Autodesk Inventor part; units mm, degrees
ref_plane "YZ Plane" through (0, 0, 0) normal (1, 0, 0) x (0, 1, 0)
ref_plane "XZ Plane" through (0, 0, 0) normal (0, 1, 0) x (-1, 0, 0)
ref_plane "XY Plane" through (0, 0, 0) normal (0, 0, 1) x (1, 0, 0)
sketch "Boceto1" plane through (0, 0, 0) normal (0, 1, 0) x (-1, 0, 0)
  line L0 (0, 0) -> (50, 0)
  line L1 (50, 0) -> (50, -65)
  line L2 (50, -65) -> (0, -65)
  line L3 (0, -65) -> (0, 0)
  line L4 (17.7, -45) -> (32.7, -45)
  line L5 (32.7, -45) -> (32.7, -20)
  line L6 (32.7, -20) -> (17.7, -20)
  line L7 (17.7, -20) -> (17.7, -45)
  line L8 (17.7, -45) -> (32.7, -20) construction
  line L9 (32.7, -45) -> (17.7, -20) construction
  line L10 (35.7, -17) -> (35.7, -48)
  line L11 (35.7, -48) -> (14.7, -48)
  line L12 (14.7, -48) -> (14.7, -17)
  line L13 (14.7, -17) -> (35.7, -17)
  line L14 (41, -1.5) -> (9, -1.5)
  line L15 (9, -1.5) -> (9, -14)
  line L16 (9, -14) -> (41, -14)
  line L17 (41, -14) -> (41, -1.5)
  line L18 (32.7, -32.5) -> (17.7, -32.5) construction
  line L19 (41, -7.75) -> (35.5, -7.75) construction
  line L20 (35.5, -7.75) -> (14.5, -7.75) construction
  line L21 (14.5, -7.75) -> (9, -7.75) construction
  circle A0 centre (35.5, -7.75) radius 1.4
  circle A1 centre (14.5, -7.75) radius 1.4
  line L22 (41, -63.5) -> (9, -63.5)
  line L23 (9, -63.5) -> (9, -51)
  line L24 (9, -51) -> (41, -51)
  line L25 (41, -51) -> (41, -63.5)
  circle A2 centre (35.5, -57.25) radius 1.4
  circle A3 centre (14.5, -57.25) radius 1.4
  line L26 (50, -32.5) -> (43.2, -32.5) construction
  line L27 (0, -32.5) -> (6.8, -32.5)
  line L28 (45.9347, 0) -> (45.9347, -14) construction
  line L29 (43.2, -32.5) -> (43.2, -14.5) construction
  line L30 (43.2, -14.5) -> (50, -14.5) construction
  circle A4 centre (43.2, -14.5) radius 1.4
  line L31 (25.2, -20) -> (25.2, -45) construction
  circle A5 centre (7.2, -14.5) radius 1.4
  circle A6 centre (35.5, -57.25) radius 1.4
  circle A7 centre (43.2, -50.5) radius 1.4
  circle A8 centre (7.2, -50.5) radius 1.4
  line L32 (35.5, -7.75) -> (14.5, -7.75)
  point P0 (25.2, -32.5)
  point P1 (25, -14)
  point P2 (25.2, -17)
  dimension "d0" = 65
  dimension "d1" = 50
  dimension "d2" = 25
  dimension "d3" = 15
  dimension "d4" = 3
  dimension "d5" = 12.5
  dimension "d6" = 32
  dimension "d7" = 3
  dimension "d8" = 5.5
  dimension "d9" = 5.5
  dimension "d10" = 2.8
  dimension "d11" = 2.8
  dimension "d12" = 6.8
  dimension "d13" = 6.8
  dimension "d14" = 14
  dimension "d15" = 2.8
  dimension "d30" = 36
  dimension "d31" = 36
  dimension "d32" = 1.5
extrude "Extrusión1" add sketch "Boceto1" along normal blind 3 contours L10 L11 L12 L13
extrude "Extrusión2" add sketch "Boceto1" against normal blind 4 contours L0 L1 L2 L3 | L17 L16 L15 L14 | L22 L23 L24 L25
extrude "Extrusión3" add sketch "Boceto1" along normal blind 2 contours L17 L16 L15 L14 | L22 L23 L24 L25
sketch "Boceto2" plane through (0, 2, 0) normal (0, 1, 0) x (1, 0, 0)
  line L0 (-41, 1.5) -> (-9, 1.5)
  line L1 (-25, 1.5) -> (-25, 14)
  line L2 (-9, 14) -> (-41, 14)
  line L3 (-20, 1.5) -> (-30, 1.5)
  line L4 (-30, 1.5) -> (-30, 14)
  line L5 (-30, 14) -> (-20, 14)
  line L6 (-20, 14) -> (-20, 1.5)
  line L7 (-20, 1.5) -> (-30, 14) construction
  line L8 (-30, 1.5) -> (-20, 14) construction
  line L9 (-32.7, 32.5) -> (-17.7, 32.5) construction
  line L10 (-41, 63.5) -> (-9, 63.5)
  line L11 (-9, 51) -> (-41, 51)
  line L12 (-30, 63.5) -> (-30, 51)
  line L13 (-20, 51) -> (-20, 63.5)
  point P0 (0, 0)
  point P1 (-25, 7.75)
  dimension "d22" = 10
extrude "Extrusión4" cut sketch "Boceto2" against normal blind 0.75
extrude "Extrusión5" add sketch "Boceto1" against normal blind 4 contours L7 L6 L5 L4 | L10 L11 L12 L13
sketch "Boceto3" plane through (0, 3, 0) normal (0, 1, 0) x (1, 0, 0)
  line L0 (-25.2, 20) -> (-25.2, 45) construction
  line L1 (-35.7, 17) -> (-14.7, 17)
  line L2 (-25.2, 17) -> (-25.2, 48)
  line L3 (-14.7, 48) -> (-35.7, 48)
  line L4 (-24.95, 17) -> (-25.45, 17)
  line L5 (-25.45, 17) -> (-25.45, 48)
  line L6 (-25.45, 48) -> (-24.95, 48)
  line L7 (-24.95, 48) -> (-24.95, 17)
  line L8 (-24.95, 17) -> (-25.45, 48) construction
  line L9 (-25.45, 17) -> (-24.95, 48) construction
  point P0 (0, 0)
  point P1 (-25.2, 32.5)
  point P2 (-24.95, 17)
  point P3 (-24.95, 48)
  point P4 (-25.45, 17)
  dimension "d27" = 0.5
extrude "Extrusión6" cut sketch "Boceto3" against normal blind 1
sketch "Boceto4" plane through (-41, 0, -1.5) normal (0, 0, 1) x (1, 0, 0)
  line L0 (16.05, 2) -> (15.55, 2)
  line L1 (21, 1.25) -> (11, 1.25)
  line L2 (-9, 0) -> (41, 0)
  line L3 (15.55, 2) -> (15.55, 3)
fillet "Empalme1" radius 2 4 edges at (-41, 1, -51) (-9, 1, -51) (-9, 1, -14) (-41, 1, -14)
equation "\"d9\" = d8"
equation "\"d13\" = d12"
properties part number "Molde 1FBR 1.0mm"
For this review, take the finished solid that the model builds, in its own axes (mm). A direction names the side the tool comes from. Round coordinates to 2 decimals unless told otherwise and drop trailing zeros. Loops run counter-clockwise (first coordinate to the right, second up) from the corner with the lowest first, then second, coordinate; pieces in that order, holes last. Notation, with made-up numbers: (-19, -35.5) - (6, -35.5) arc R21 ccw to (6, -14.5) - close; hole circle Ø11 at (-31, 13.5). An arc over 180 degrees is marked (long way). One line per question, with ' | ' between items.
Q1. Take a section at A-A (z = -57.25). Give the boundary of the cut face in (x, y).
Taken from the geometry:
outline: (-50, -4) - (-36.9, -4) - (-36.9, 2) - (-41, 2) - (-41, 0) - (-50, 0) - close; (-34.1, -4) - (-15.9, -4) - (-15.9, 2) - (-20, 2) - (-20, 1.25) - (-30, 1.25) - (-30, 2) - (-34.1, 2) - close; (-13.1, -4) - (0, -4) - (0, 0) - (-9, 0) - (-9, 2) - (-13.1, 2) - close
Q2. Take a section at B-B (y = -2.25). State how many separate pieces and enclosed holes the cut face has, and give its area (3 significant figures).
Taken from the geometry:
separate pieces: 1 | enclosed holes: 8 | area: 3,200 mm²
Q3. Take a section at C-C (x = -27). Give the boundary of the cut face in (y, z), and give its area (3 significant figures).
Taken from the geometry:
outline: (-4, -65) - (0, -65) - (0, -63.5) - (1.25, -63.5) - (1.25, -51) - (0, -51) - (0, -48) - (3, -48) - (3, -45) - (0, -45) - (0, -20) - (3, -20) - (3, -17) - (0, -17) - (0, -14) - (1.25, -14) - (1.25, -1.5) - (0, -1.5) - (0, 0) - (-4, 0) - close | area: 309 mm²
Q4. For pin 1 (1.6 mm diameter, centred on x = -18, y = 1, fed in from -Z); pin 2 (1.5 mm diameter, centred on y = 1.5, z = -30, fed in from -X); pin 3 (3.5 mm diameter, centred on x = -13.5, z = -9.5, fed in from +Y); pin 4 (4 mm diameter, centred on y = 1.5, z = -55, fed in from -X), all flat-tipped, find the tip position at first contact; note any pin that passes through.
Taken from the geometry:
pin 1: stops at z = -63.5 | pin 2: stops at x = -35.7 | pin 3: stops at y = 2 | pin 4: stops at x = -50
Q5. The part is to be moulded in two halves that separate along X. For faces 1 (the cylindrical face through (-7.95, -1.97, -13.32)), 2 (the flat face through (-35, 2, -6)), 3 (the cylindrical face through (-9.6, 1.01, -51.57)), say which applies: released by +X, released by -X, zero draft, split by the parting line, or undercut.
Taken from the geometry:
face 1: undercut | face 2: zero draft | face 3: released by +X
Q6. Take a section at D-D (z = -29.5). Give the boundary of the cut face in (x, y).
Taken from the geometry:
outline: (-50, -4) - (0, -4) - (0, 0) - (-14.7, 0) - (-14.7, 3) - (-17.7, 3) - (-17.7, 0) - (-32.7, 0) - (-32.7, 3) - (-35.7, 3) - (-35.7, 0) - (-50, 0) - close
Q7. For line 1 along Z through (x, y) = (-7.2, -2.45); line 2 along Z through (x, y) = (-19, 0.5); line 3 along Z through (x, y) = (-14.5, -0.5), list the stretches that pass through material, from the lowest coordinate up. Write a range as [from, to].
Taken from the geometry:
line 1: z = [-65, -51.9], [-49.1, -15.9], [-13.1, 0] | line 2: z = [-63.5, -51], [-48, -45], [-20, -17], [-14, -1.5] | line 3: z = [-65, -58.65], [-55.85, -9.15], [-6.35, 0]
Q8. Tool access review of faces 4 (the flat face through (-32.7, 1, -33)), 5 (the flat face through (-25, 1.25, -57)), 6 (the flat face through (-34, 2, -56)), 7 (the flat face through (-9, 1, -58)): name each direction out of +Z, -Z, +X, -X, +Y, -Y from which nothing blocks a thin tool from reaching the whole face with its end or side.
Taken from the geometry:
face 4: +Y | face 5: -Z, +Y | face 6: -Z, +X, -X, +Y | face 7: +Z, -Z, +X, +Y
